Geometry check sheet. Reference: the model listing, model coordinates, mm. A direction names the side the tool comes from. Round coordinates to 2 decimals unless told otherwise and drop trailing zeros. Order: outer loops, then holes, each group sorted by start corner. A loop starts at its lowest first (then second) coordinate and runs counter-clockwise, first axis right, second up. Notation, with made-up numbers: (-8, -39.5) - (26, -39.5) arc R26 ccw to (26, -22.5) - close; hole circle Ø11 at (5, 59.25). An arc over 180 degrees is marked (long way). Return JSON: item names as keys, results as strings. Group by question number.
Q1. Material ranges on line 1 along Y through (x, z) = (12.5, 38.1) (3 decimals); line 2 along Z through (x, y) = (13, 69.85) (3 decimals); line 3 along Y through (x, z) = (13, 18.5), recorded low to high.
Q2. Sectioned sample at C-C, the plane x = 4. Record the cut outline in (y, z), then the cut area to 3 significant figures.
Q3. Sectioned sample at B-B, the plane z = 8.5. Record the cut outline in (x, y).
Q4. Gauge pin test, flat ends, axial feed: pin 1 Ø3 at (x, z) = (3.5, 21) entering from +Y; pin 2 Ø12.5 at (y, z) = (20, 36) entering from +X; pin 3 Ø5 at (x, y) = (16.5, 63) entering from -Z; pin 4 Ø1 at (y, z) = (52.5, 52) entering from +X. Record the tip position at first contact, or that the pin passes through.
Q5. Sectioned sample at D-D, the plane y = 48. Record the cut outline in (x, z) (3 decimals).
Q6. Draft check along Z on faces 5 (the cylindrical face through (12.66, 72.95, 38.79)), 6 (the flat face through (22, 6.35, 38)), 7 (the flat face through (13, 13, 76.2)). Enter one of: pulls with the +Z half, pulls with the -Z half, needs draft (parallel to the pull), parting line crosses it, or undercut.
Q7. Tool access check on faces 1 (the flat face through (15.875, 57, 38)), 2 (the flat face through (13, 51, 50.8)), 3 (the flat face through (3, 6.35, 38)), 4 (the flat face through (13, 51, 25.4)). Record the directions out of +Z, -Z, +X, -X, +Y, -Y that give a thin tool (end or side, any length) a straight path to the whole face; none if there is none.
Autodesk Inventor part; units mm, degrees
ref_plane "YZ Plane" through (0, 0, 0) normal (1, 0, 0) x (0, 1, 0)
ref_plane "XZ Plane" through (0, 0, 0) normal (0, 1, 0) x (-1, 0, 0)
ref_plane "XY Plane" through (0, 0, 0) normal (0, 0, 1) x (1, 0, 0)
sketch "Sketch1" plane through (0, 0, 0) normal (0, 0, 1) x (1, 0, 0)
  line L0 (0, 0) -> (25.4, 0)
  line L1 (25.4, 0) -> (25.4, 6.35)
  line L2 (25.4, 6.35) -> (19.05, 6.35)
  line L3 (19.05, 6.35) -> (19.05, 31.75)
  line L4 (19.05, 31.75) -> (6.35, 31.75)
  line L5 (6.35, 31.75) -> (6.35, 6.35)
  line L6 (6.35, 6.35) -> (0, 6.35)
  line L7 (0, 6.35) -> (0, 0)
  dimension "d0" = 12.7
  dimension "d1" = 6.35
  dimension "d2" = 6.35
  dimension "d3" = 6.35
  dimension "d4" = 25.4
extrude "Extrusion1" add sketch "Sketch1" along normal blind 76.2
sketch "Sketch2" plane through (6.35, 31.75, 0) normal (0, 1, 0) x (1, 0, 0)
  line L0 (9.525, -50.8) -> (3.175, -50.8)
  line L1 (3.175, -50.8) -> (3.175, -25.4)
  line L2 (3.175, -25.4) -> (9.525, -25.4)
  line L3 (9.525, -25.4) -> (9.525, -50.8)
  line L4 (0, 0) -> (0, -76.2)
  line L5 (12.7, 0) -> (12.7, -76.2)
  line L6 (12.7, -76.2) -> (0, -76.2)
  line L7 (12.7, 0) -> (0, 0)
  point P0 (-6.35, 0)
  dimension "d7" = 12.7
  dimension "d8" = 3.175
  dimension "d9" = 3.175
  dimension "d10" = 6.35
  dimension "d11" = 76.2
  dimension "d12" = 25.4
  dimension "d13" = 25.4
extrude "Extrusion2" add sketch "Sketch2" along normal blind 50.8 contours L0 L1 L2 L3
fillet "Fillet1" radius 12.7 2 edges at (12.7, 82.55, 50.8) (12.7, 82.55, 25.4)
hole "Hole1" at (15.875, 69.85, 38.1) direction (-1, 0, 0) diameter 6.35 end through all
properties part number "slider"
Reply:
{
 "1": {"line 1": "0 to 66.675, 73.025 to 82.55", "line 2": "25.4 to 34.925, 41.275 to 50.8", "line 3": "0 to 31.75"},
 "2": {"outline": "(0, 0) - (6.35, 0) - (6.35, 76.2) - (0, 76.2) - close", "area": "484 mm^2"},
 "3": {"outline": "(0, 0) - (25.4, 0) - (25.4, 6.35) - (19.05, 6.35) - (19.05, 31.75) - (6.35, 31.75) - (6.35, 6.35) - (0, 6.35) - close"},
 "4": {"pin 1": "y = 6.35", "pin 2": "x = 19.05", "pin 3": "z = 25.4", "pin 4": "through"},
 "5": {"outline": "(9.525, 25.4) - (15.875, 25.4) - (15.875, 50.8) - (9.525, 50.8) - close"},
 "6": {"face 5": "undercut", "face 6": "needs draft", "face 7": "pulls with the +Z half"},
 "7": {"face 1": "+Z, -Z, +X, +Y", "face 2": "+Z, +X, -X, +Y", "face 3": "+Z, -Z, -X, +Y", "face 4": "-Z, +X, -X, +Y"}
}
